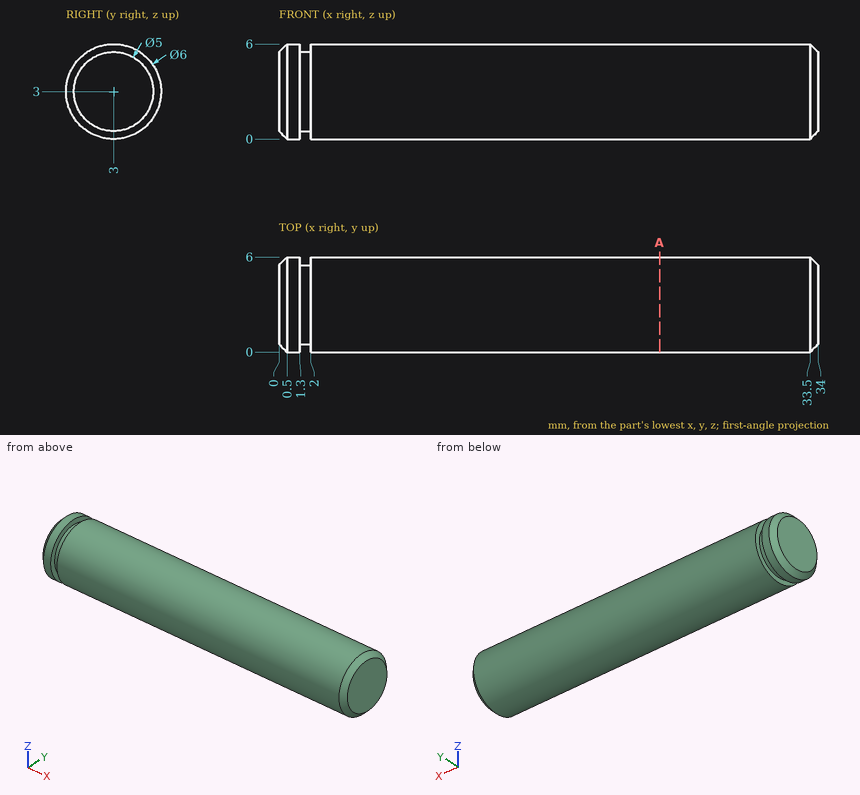
The drawing under review shows one solid part. Ordinate dimensions are in mm from its lowest x, y, z. Round coordinates to 2 decimals unless told otherwise and drop trailing zeros. Loops run counter-clockwise (first coordinate to the right, second up) from the corner with the lowest first, then second, coordinate; pieces in that order, holes last. Notation, with made-up numbers: (58, 57) -> (81, 57) arc R25 ccw to (81, 79) -> close; hole circle Ø2 at (53.25, 50). An arc over 180 degrees is marked (long way). One line per question, with ' | ' between items. Start each with the question number.
Item 1: Wall thickness on line 1 along X through (y, z) = (4.85, 5.2); line 2 along Y through (x, z) = (6.5, 4.65); line 3 along X through (y, z) = (4.65, 0.8): over which ranges is each line inside the solid? List them lowest first. Write a range as [from, to].
Item 2: Add section A-A, the plane x = 24. Write out the cut boundary in (y, z).
Item 3: For pin 1 (3 mm diameter, centred on x = 9, y = 5, fed in from +Z); pin 2 (1 mm diameter, centred on x = 26.5, z = 1.5, fed in from +Y), all flat-tipped, find the tip position at first contact; note any pin that passes through.
Return value:
1) line 1: x = [0.37, 1.3], [2, 33.63] | line 2: y = [0.49, 5.51] | line 3: x = [0.25, 1.3], [2, 33.75]
2) outline: circle Ø6 at (3, 3)
3) pin 1: stops at z = 5.96 | pin 2: stops at y = 5.83
